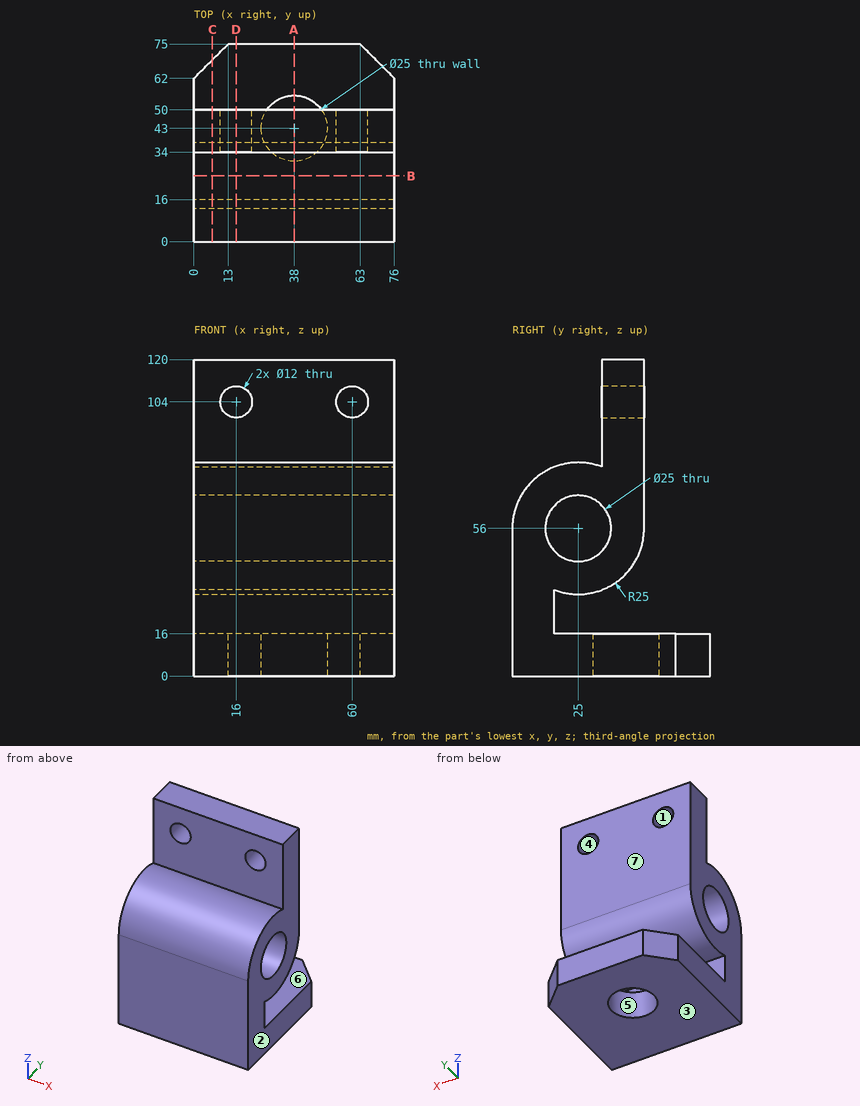
Could you check a few things on this drawing? It's one solid part, dimensions in mm from its lowest x, y, z. A direction names the side the tool comes from. Coordinates: 2 decimals unless noted, no trailing zeros. Order: outer loops, then holes, each group sorted by start corner. A loop starts at its lowest first (then second) coordinate and runs counter-clockwise, first axis right, second up. Notation, with made-up numbers: (-12, -14) - (30, -14) arc R30 cw to (30, 17) - close; hole circle Ø11 at (81.5, -0.75). An arc over 180 degrees is marked (long way). Answer as a JSON object with one key per item and string values. Group by question number.
Q1. Imagine slicing it at B-B (y = 25). Please give me the cut outline in (x, z), and give its area (3 significant figures).
Q2. Imagine slicing it at A-A (x = 38). Please give me the cut outline in (y, z), and give its area (3 significant figures).
Q3. On a 3-axis mill with a long thin cutter (end or side, diameter ignored), from which of +Z, -Z, +X, -X, +Y, -Y can I reach the whole of each face in a straight line? I mean the marked faces 5, 6 and 7. Say none if no direction works.
Q4. Imagine slicing it at C-C (x = 7). Please give me the cut outline in (y, z).
Q5. Imagine slicing it at D-D (x = 16). Please give me the cut outline in (y, z).
Q6. Will these pins go through, and if not, where does the flat tip stop? P1, Ø8, axis at x = 44, y = 41, coming from the -Z side; P2, Ø5, axis at y = 31.5, z = 43, coming from the -X side; P3, Ø19, axis at x = 60, z = 104, coming from the +Y side; P4, Ø2, axis at x = 15.5, z = 52.5, coming from the +Y side.
Q7. We'd pull the mould along X, two halves only. Please class the marked faces 1, 2, 3 and 4: +X half, -X half, draft (parallel to the pull), parting line (faces both ways), or undercut.
Q8. I need wall thicknesses on line 1 (Y direction, x = 38, z = 4); line 2 (Z direction, x = 25.5, y = 32); line 3 (Y direction, x = 36.5, z = 20.5). Which ranges of each line are inside material? Lowest first, please. Write a range as from..to.
Determined:
{
 "1": {"outline": "(0, 0) - (76, 0) - (76, 16) - (0, 16) - close; (0, 31) - (76, 31) - (76, 43.5) - (0, 43.5) - close; (0, 68.5) - (76, 68.5) - (76, 81) - (0, 81) - close", "area": "3,120 mm2"},
 "2": {"outline": "(0, 0) - (30.5, 0) - (30.5, 16) - (16, 16) - (16, 32.68) arc R25 ccw to (50, 56) - (50, 120) - (34, 120) - (34, 79.32) arc R25 ccw to (0, 56) - close; (55.5, 0) - (75, 0) - (75, 16) - (55.5, 16) - close; hole circle Ø25 at (25, 56)", "area": "3,390 mm2"},
 "3": {"face 5": "-Z", "face 6": "+X, -X, +Y", "face 7": "+Z, +X, -X, +Y"},
 "4": {"outline": "(0, 0) - (69, 0) - (69, 16) - (16, 16) - (16, 32.68) arc R25 ccw to (50, 56) - (50, 120) - (34, 120) - (34, 79.32) arc R25 ccw to (0, 56) - close; hole circle Ø25 at (25, 56)"},
 "5": {"outline": "(0, 0) - (75, 0) - (75, 16) - (16, 16) - (16, 32.68) arc R25 ccw to (50, 56) - (50, 98) - (34, 98) - (34, 79.32) arc R25 ccw to (0, 56) - close; (34, 110) - (50, 110) - (50, 120) - (34, 120) - close; hole circle Ø25 at (25, 56)"},
 "6": {"P1": "stops at z = 34.07", "P2": "stops at x = 0", "P3": "stops at y = 50", "P4": "stops at y = 49.87"},
 "7": {"face 1": "undercut", "face 2": "+X half", "face 3": "draft", "face 4": "undercut"},
 "8": {"line 1": "y = 0..30.5, 55.5..75", "line 2": "z = 0..16, 32..45.64, 66.36..80", "line 3": "y = 0..16"}
}
